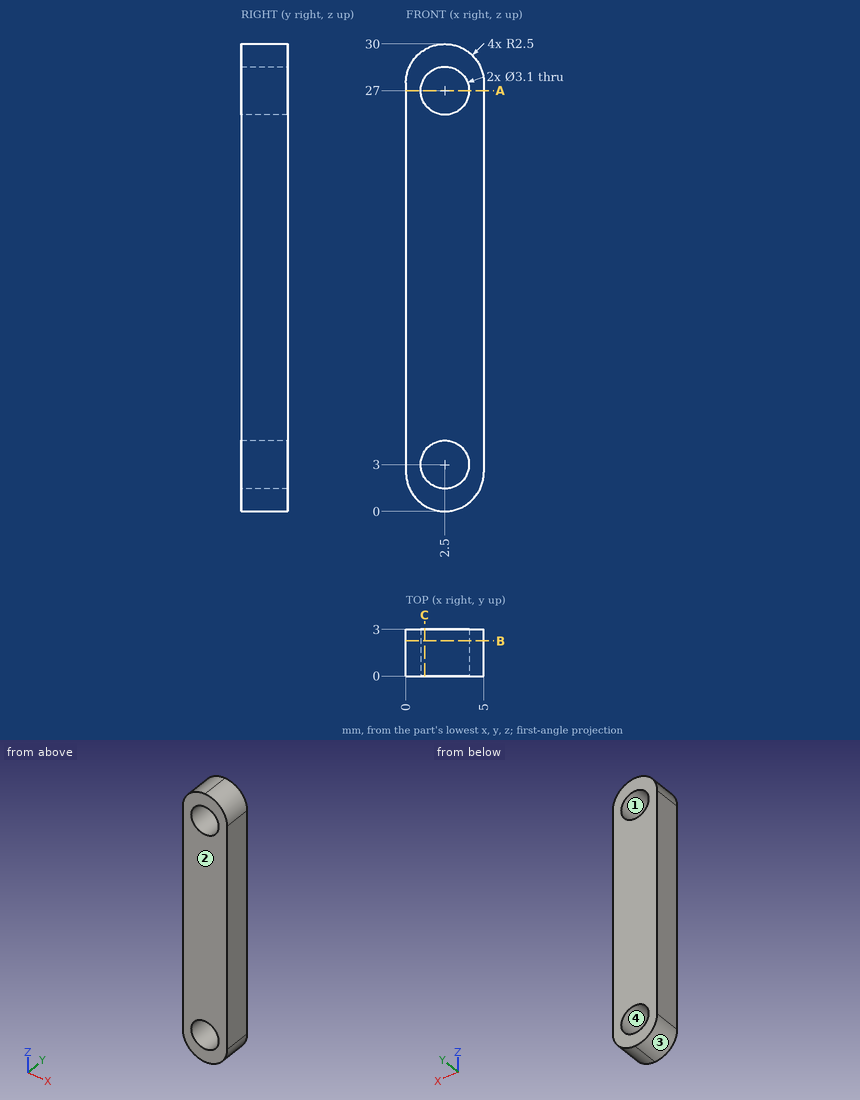
Source: three-view drawing plus pictorial views. Frame: mm from the lowest corner of the part. Give positions to 0.01 mm unless a question says otherwise; leave off trailing zeros. Order: outer loops, then holes, each group sorted by start corner. A loop starts at its lowest first (then second) coordinate and runs counter-clockwise, first axis right, second up. Notation, with made-up numbers: (-17.5, 44.5) -> (40.5, 44.5) arc R14 ccw to (40.5, 54.5) -> close; hole circle Ø11 at (55.25, 62.5). An arc over 180 degrees is marked (long way). Write each question's results on one line, items separated by ' | '. Start each with the question number.
Item 1: Cut plane A-A on z = 27. Return the cut outline in (x, y), then the cut area to 3 significant figures.
Item 2: Contact query for flat-ended pins moving along their axis: P1, Ø3, axis at x = 1, z = 7, coming from the -Y side; P2, Ø1, axis at x = 3.5, y = 2, coming from the +Z side. Output: stop coordinate, or through.
Item 3: Cut plane B-B on y = 2.25. Give the number of separate pieces and of enclosed holes in the cut face, then the cut area to 3 significant figures.
Item 4: Cut plane C-C on x = 1.2. Return the cut outline in (y, z).
Item 5: Line query: line 1 (Z direction, x = 1.65, y = 1.65); line 2 (Z direction, x = 1.9, y = 0.85); line 3 (X direction, y = 2.45, z = 27). Output: solid intervals per line, ascending.
Item 6: Mould query, pull axis Z, two halves, no side actions, for the marked faces 1, 2, 3 and 4. Classes: pulls with the +Z half, pulls with the -Z half, needs draft (parallel to the pull), parting line crosses it, or undercut.
Established:
1) outline: (0, 0) -> (0.95, 0) -> (0.95, 3) -> (0, 3) -> close; (4.05, 0) -> (5, 0) -> (5, 3) -> (4.05, 3) -> close | area: 5.70 mm^2
2) P1: y = 0 | P2: z = 29.95
3) separate pieces: 1 | enclosed holes: 2 | area: 130 mm^2
4) outline: (0, 0.36) -> (3, 0.36) -> (3, 2.16) -> (0, 2.16) -> close; (0, 3.84) -> (3, 3.84) -> (3, 26.16) -> (0, 26.16) -> close; (0, 27.84) -> (3, 27.84) -> (3, 29.64) -> (0, 29.64) -> close
5) line 1: 0.15 to 1.7, 4.3 to 25.7, 28.3 to 29.85 | line 2: 0.07 to 1.57, 4.43 to 25.57, 28.43 to 29.93 | line 3: 0 to 0.95, 4.05 to 5
6) face 1: undercut | face 2: needs draft | face 3: pulls with the -Z half | face 4: undercut
